```python
from build123d import *

# Parameters (mm, degrees)
SKETCH1_R           = 19.05
BOSS_EXTRUDE1_DEPTH = 2.54
SKETCH2_R           = 15.875
BOSS_EXTRUDE2_DEPTH = 7.62
CUT_EXTRUDE1_REACH  = 14.7
SKETCH4_R           = 3.175
CUT_EXTRUDE2_REACH  = 14.7
SKETCH5_R           = 1.5875


with BuildPart() as part:
    # Sketch1 → Boss-Extrude1 (new body)
    with BuildSketch(Plane.XY):
        Circle(SKETCH1_R)
    boss_extrude1 = extrude(amount=BOSS_EXTRUDE1_DEPTH)

    # Sketch2 → Boss-Extrude2 (add)
    with BuildSketch(Plane.XY.offset(2.54)):
        Circle(SKETCH2_R)
    extrude(amount=BOSS_EXTRUDE2_DEPTH)

    # Mirror1: Boss-Extrude1 across plane
    add(boss_extrude1.mirror(Plane.XY.offset(6.35)))

    # Sketch4 → Cut-Extrude1 (cut, up to next)
    with BuildSketch(Plane.XY.offset(12.7), mode=Mode.PRIVATE) as cut_extrude1_sk1:
        Circle(SKETCH4_R)
    cut_extrude1_tool1 = extrude(cut_extrude1_sk1.sketch, amount=-CUT_EXTRUDE1_REACH, mode=Mode.PRIVATE) & part.part
    add(cut_extrude1_tool1.solids().sort_by_distance((0, 0, 12.7))[0], mode=Mode.SUBTRACT)

    # Sketch5 → Cut-Extrude2 (cut, up to next)
    with BuildSketch(Plane(origin=(0, 0, 0), x_dir=(-1, 0, 0), z_dir=(0, 0, -1)), mode=Mode.PRIVATE) as cut_extrude2_sk1:
        with Locations((0, 12.7)):
            Circle(SKETCH5_R)
    cut_extrude2_tool1 = extrude(cut_extrude2_sk1.sketch, amount=-CUT_EXTRUDE2_REACH, mode=Mode.PRIVATE) & part.part
    add(cut_extrude2_tool1.solids().sort_by_distance((0, 12.7, 0))[0], mode=Mode.SUBTRACT)
    # Sketch5 → Cut-Extrude2 (cut, up to next)
    with BuildSketch(Plane(origin=(0, 0, 0), x_dir=(-1, 0, 0), z_dir=(0, 0, -1)), mode=Mode.PRIVATE) as cut_extrude2_sk2:
        with Locations((12.7, 0)):
            Circle(SKETCH5_R)
    cut_extrude2_tool2 = extrude(cut_extrude2_sk2.sketch, amount=-CUT_EXTRUDE2_REACH, mode=Mode.PRIVATE) & part.part
    add(cut_extrude2_tool2.solids().sort_by_distance((-12.7, 0, 0))[0], mode=Mode.SUBTRACT)
    # Sketch5 → Cut-Extrude2 (cut, up to next)
    with BuildSketch(Plane(origin=(0, 0, 0), x_dir=(-1, 0, 0), z_dir=(0, 0, -1)), mode=Mode.PRIVATE) as cut_extrude2_sk3:
        with Locations((0, -12.7)):
            Circle(SKETCH5_R)
    cut_extrude2_tool3 = extrude(cut_extrude2_sk3.sketch, amount=-CUT_EXTRUDE2_REACH, mode=Mode.PRIVATE) & part.part
    add(cut_extrude2_tool3.solids().sort_by_distance((0, -12.7, 0))[0], mode=Mode.SUBTRACT)
    # Sketch5 → Cut-Extrude2 (cut, up to next)
    with BuildSketch(Plane(origin=(0, 0, 0), x_dir=(-1, 0, 0), z_dir=(0, 0, -1)), mode=Mode.PRIVATE) as cut_extrude2_sk4:
        with Locations((-12.7, 0)):
            Circle(SKETCH5_R)
    cut_extrude2_tool4 = extrude(cut_extrude2_sk4.sketch, amount=-CUT_EXTRUDE2_REACH, mode=Mode.PRIVATE) & part.part
    add(cut_extrude2_tool4.solids().sort_by_distance((12.7, 0, 0))[0], mode=Mode.SUBTRACT)


solid = part.part
```
Work out the finished part from the listing and answer in its coordinate system (mm). A direction names the side the tool comes from. Round coordinates to 2 decimals unless told otherwise and drop trailing zeros. Loops run counter-clockwise (first coordinate to the right, second up) from the corner with the lowest first, then second, coordinate; pieces in that order, holes last. Notation, with made-up numbers: (59.5, 37.5) -> (100.5, 37.5) arc R13 ccw to (100.5, 56.5) -> close; hole circle Ø11 at (-9, -19.75). An arc over 180 degrees is marked (long way). Write each question's results on one line, items separated by ' | '. Start each with the question number.
1. For a pull along X with two mould halves and no side action, classify faces 3 (the face through (0.207, 14.274, 6.261)), 4 (the face through (-4, 16, 2.54)), 5 (the face through (-3.441, -15.497, 6.297)) as +X half, -X half, draft (parallel to the pull), parting line (faces both ways), or undercut.
2. Section D-D (x = -12) is taken. Determine the outline of the cut face in (y, z), plus the area to 3 significant figures.
3. A tool of negligible diameter and unlimited length cuts with its end or side. For faces 1 (the face through (-4, 16, 10.16)), 2 (the face through (-15.12, -11.59, 1.25)), from which of +Z, -Z, +X, -X, +Y, -Y can it reach the whole face along a straight path? Write none if from no direction.
4. Find the intervals of material crossed by probe 1 along Y at (x, z) = (0, 4.25) (1 decimal); probe 2 along Z at (x, y) = (-17, -4.5); probe 3 along Y at (x, z) = (12.7, 3.25) (1 decimal), in increasing order. Write a range as from..to.
5. Given pin 1 Ø3 at (x, y) = (-12.7, 0) entering from -Z; pin 2 Ø2 at (x, z) = (13.5, 10.5) entering from +Y; pin 3 Ø3.5 at (x, y) = (12.7, 0) entering from +Z; pin 4 Ø6 at (x, z) = (5.5, 11.5) entering from +Y, each flat-ended and moving along its own axis, determine where each tip first touches the part or whether it passes through.
6. Section A-A (y = 0) is taken. State how many separate pieces and enclosed holes the cut face has, plus the area to 3 significant figures.
Evaluation:
1) face 3: undercut | face 4: draft | face 5: parting line
2) outline: (-14.8, 0) -> (-1.42, 0) -> (-1.42, 12.7) -> (-14.8, 12.7) -> (-14.8, 10.16) -> (-10.39, 10.16) -> (-10.39, 2.54) -> (-14.8, 2.54) -> close; (1.42, 0) -> (14.8, 0) -> (14.8, 2.54) -> (10.39, 2.54) -> (10.39, 10.16) -> (14.8, 10.16) -> (14.8, 12.7) -> (1.42, 12.7) -> close | area: 273 mm2
3) face 1: none | face 2: +Z, -Z
4) probe 1: y = -15.9..-14.3, -11.1..-3.2, 3.2..11.1, 14.3..15.9 | probe 2: z = 0..2.54, 10.16..12.7 | probe 3: y = -9.5..-1.6, 1.6..9.5
5) pin 1: passes through | pin 2: stops at y = 14.38 | pin 3: stops at z = 12.7 | pin 4: stops at y = 18.89
6) separate pieces: 4 | enclosed holes: 0 | area: 274 mm2
